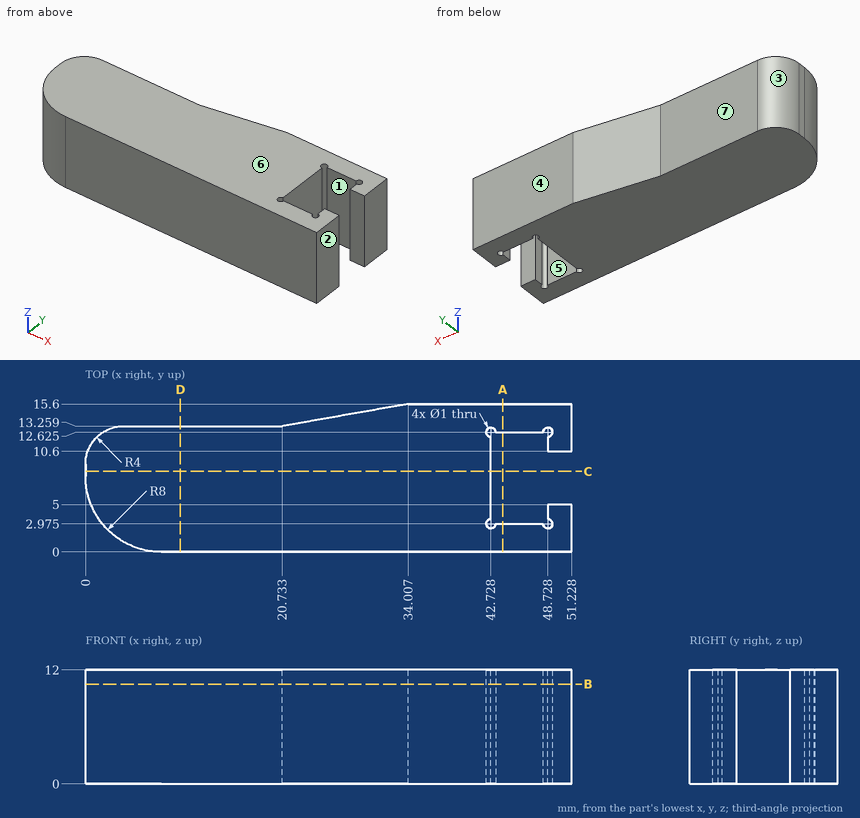
For this review, use the dimensioned drawing (mm, ordinates from the lowest corner) and the shaded views. A direction names the side the tool comes from. Round coordinates to 2 decimals unless told otherwise and drop trailing zeros. Order: outer loops, then holes, each group sorted by start corner. A loop starts at its lowest first (then second) coordinate and runs counter-clockwise, first axis right, second up. Notation, with made-up numbers: (77.25, -27.75) -> (130.25, -27.75) arc R21 cw to (130.25, 1.25) -> close; hole circle Ø4 at (25.5, 18.5). An arc over 180 degrees is marked (long way). Write item = value, one per line. Start each with the question number.
Item 1: Consider section A-A on x = 44. Write out the cut boundary in (y, z) (1 decimal).
Item 2: For the marked faces 5, 6 and 7, list the 3-axis set-ups (+Z, -Z, +X, -X, +Y, -Y) from which the entire face can be reached by the end or side of a thin tool; tool diameter is ignored.
Item 3: Mouldability with a two-part tool opening along X and no side actions: class the marked faces 1, 2, 3 and 4 as released by +X, released by -X, zero draft, split by the parting line, or undercut.
Item 4: Clearance check with flat-ended pins moving along their axes: pin 1 Ø0.5 at (y, z) = (11, 6) entering from -X; pin 2 Ø0.8 at (y, z) = (4, 5.5) entering from -X (1 decimal); pin 3 Ø3 at (y, z) = (13, 6.5) entering from -X (1 decimal). State where each tip first meets the part, or that it passes through.
Item 5: Consider section C-C on y = 8.5. Write out the cut boundary in (x, z).
Item 6: For line 1 along Y through (x, z) = (45, 11) (1 decimal); line 2 along Y through (x, z) = (49, 3) (1 decimal); line 3 along Y through (x, z) = (19.5, 7.5), list the stretches that pass through material, from the lowest coordinate up.
Item 7: Consider section D-D on x = 10. Write out the cut boundary in (y, z).
Item 8: Consider section B-B on z = 10.5. Write out the cut boundary in (x, y) (1 decimal).
Conclusion:
q1.outline = (0, 0) -> (3, 0) -> (3, 12) -> (0, 12) -> close; (12.6, 0) -> (15.6, 0) -> (15.6, 12) -> (12.6, 12) -> close
q2.face_5 = +Z, -Z
q2.face_6 = +Z, +X, -X, +Y, -Y
q2.face_7 = +Z, -Z, -X, +Y
q3.face_1 = undercut
q3.face_2 = released by +X
q3.face_3 = released by -X
q3.face_4 = zero draft
q4.pin_1 = 0.29
q4.pin_2 = 0.9
q4.pin_3 = 0.7
q5.outline = (0, 0) -> (42.73, 0) -> (42.73, 12) -> (0, 12) -> close
q6.line_1 = 0 to 3, 12.6 to 15.6
q6.line_2 = 0 to 2.6, 3.4 to 5, 10.6 to 12.2, 13 to 15.6
q6.line_3 = 0 to 13.26
q7.outline = (0, 0) -> (13.26, 0) -> (13.26, 12) -> (0, 12) -> close
q8.outline = (0, 8) arc R8 ccw to (8, 0) -> (51.2, 0) -> (51.2, 5) -> (48.7, 5) -> (48.7, 3.5) arc R0.5 cw (long way) to (48.2, 3) -> (43.2, 3) arc R0.5 cw (long way) to (42.7, 3.5) -> (42.7, 12.1) arc R0.5 cw (long way) to (43.2, 12.6) -> (48.2, 12.6) arc R0.5 cw (long way) to (48.7, 12.1) -> (48.7, 10.6) -> (51.2, 10.6) -> (51.2, 15.6) -> (34, 15.6) -> (20.7, 13.3) -> (4, 13.3) arc R4 ccw to (0, 9.3) -> close
